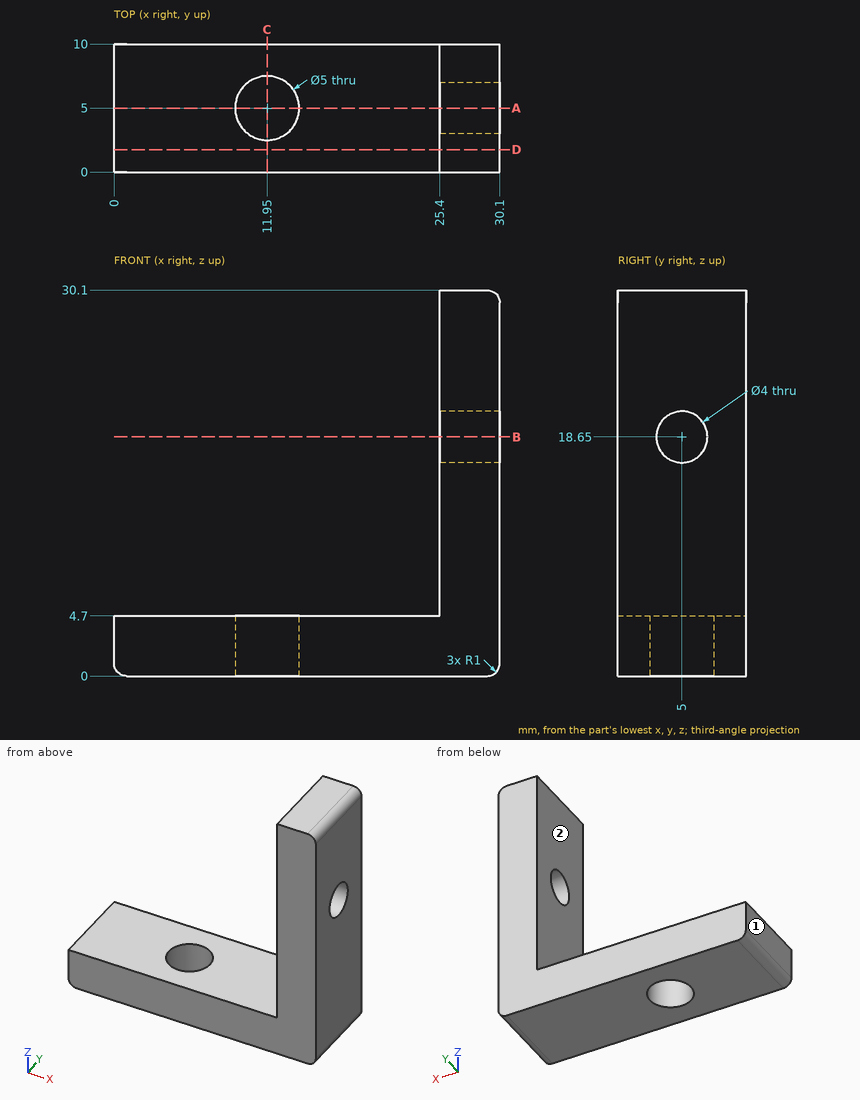
Can you work these out from the drawing? Everything is in mm from the part's minimum corner. A direction names the side the tool comes from. Give positions to 0.01 mm unless a question says otherwise; leave off trailing zeros. Loops run counter-clockwise (first coordinate to the right, second up) from the corner with the lowest first, then second, coordinate; pieces in that order, holes last. Notation, with made-up numbers: (47.5, -11) -> (67.5, -11) arc R20 cw to (67.5, -6) -> close; hole circle Ø2 at (-34, 26.5). An arc over 180 degrees is marked (long way). Return JSON: item names as keys, results as strings.
Q1. I want a section at A-A, the plane y = 5. List the corners of the cut face in (x, z) for me.
Checks:
{"outline": "(0, 1) arc R1 ccw to (1, 0) -> (9.45, 0) -> (9.45, 4.7) -> (0, 4.7) -> close; (14.45, 0) -> (29.1, 0) arc R1 ccw to (30.1, 1) -> (30.1, 16.65) -> (25.4, 16.65) -> (25.4, 4.7) -> (14.45, 4.7) -> close; (25.4, 20.65) -> (30.1, 20.65) -> (30.1, 29.1) arc R1 ccw to (29.1, 30.1) -> (25.4, 30.1) -> close"}
Q2. On a 3-axis mill with a long thin cutter (end or side, diameter ignored), from which of +Z, -Z, +X, -X, +Y, -Y can I reach the whole of each face in a straight line? I mean the marked faces 1 and 2. Say none if no direction works.
Checks:
{"face 1": "+Z, -Z, -X, +Y, -Y", "face 2": "+Z, -X, +Y, -Y"}
Q3. I want a section at C-C, the plane x = 11.95. List the corners of the cut face in (y, z) for me, then the cut area to 3 significant figures.
Checks:
{"outline": "(0, 0) -> (2.5, 0) -> (2.5, 4.7) -> (0, 4.7) -> close; (7.5, 0) -> (10, 0) -> (10, 4.7) -> (7.5, 4.7) -> close", "area": "23.5 mm2"}
Q4. I want a section at D-D, the plane y = 1.75. List the corners of the cut face in (x, z) for me.
Checks:
{"outline": "(0, 1) arc R1 ccw to (1, 0) -> (29.1, 0) arc R1 ccw to (30.1, 1) -> (30.1, 29.1) arc R1 ccw to (29.1, 30.1) -> (25.4, 30.1) -> (25.4, 4.7) -> (0, 4.7) -> close"}
Q5. I need wall thicknesses on probe 1 along Z at (x, y) = (20.5, 2); probe 2 along X at (y, z) = (6.5, 21); probe 3 along Y at (x, z) = (11, 2). Which ranges of each line are inside material? Lowest first, please.
Checks:
{"probe 1": "z = 0 to 4.7", "probe 2": "x = 25.4 to 30.1", "probe 3": "y = 0 to 2.69, 7.31 to 10"}
Q6. I want a section at B-B, the plane z = 18.65. List the corners of the cut face in (x, y) for me.
Checks:
{"outline": "(25.4, 0) -> (30.1, 0) -> (30.1, 3) -> (25.4, 3) -> close; (25.4, 7) -> (30.1, 7) -> (30.1, 10) -> (25.4, 10) -> close"}
Q7. For pin 1 Ø6 at (x, y) = (11.95, 5) entering from +Z; pin 2 Ø5 at (y, z) = (4.5, 14.5) entering from -X, each with a flat end and sliding along its axis, tell me the tip position at first contact or that it passes through.
Checks:
{"pin 1": "stops at z = 4.7", "pin 2": "stops at x = 25.4"}
